Source: three-view drawing plus pictorial views. Frame: mm from the lowest corner of the part. A direction names the side the tool comes from. Coordinates: 2 decimals unless noted, no trailing zeros. Order: outer loops, then holes, each group sorted by start corner. A loop starts at its lowest first (then second) coordinate and runs counter-clockwise, first axis right, second up. Notation, with made-up numbers: (85, 76.25) -> (94, 76.25) arc R18 ccw to (94, 95.25) -> close; hole circle Ø11 at (-11.75, 37.5). An arc over 180 degrees is marked (long way). One line per question, with ' | ' between items.
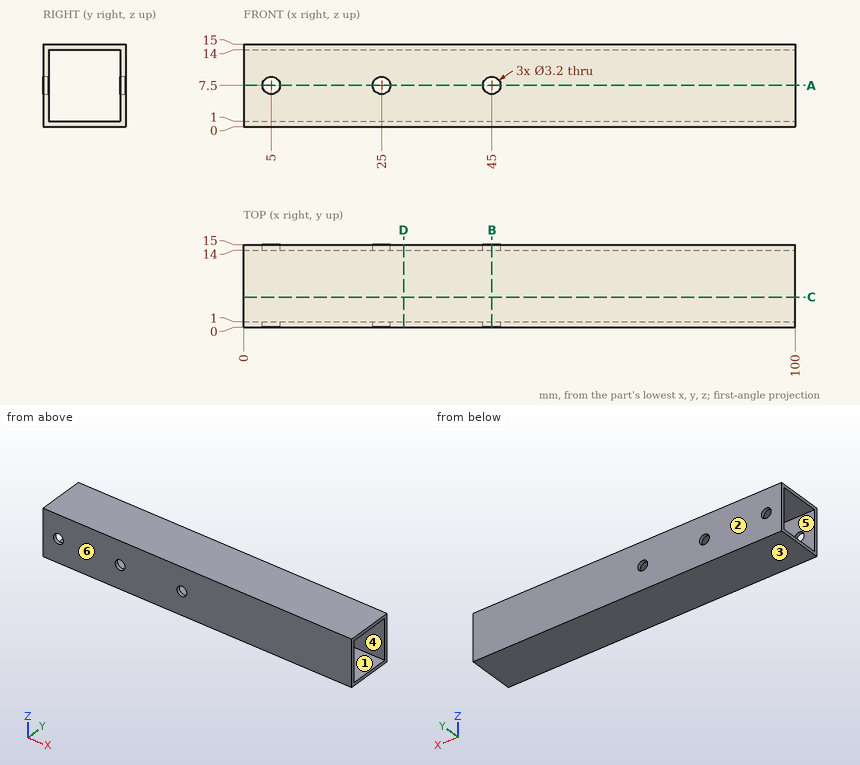
1. Access query for the marked faces 5 and 6. Directions: +Z, -Z, +X, -X, +Y, -Y. A direction counts if a zero-diameter tool reaches every point of the face in a straight line with its end or side. Return the directions, or none.
Recorded:
face 5: +X, -X | face 6: +Z, -Z, +X, -X, -Y
2. Pin query (flat end, axial travel): pin 1 Ø1.9 at (x, z) = (5, 7.5) entering from +Y; pin 2 Ø4 at (x, z) = (32.5, 3.5) entering from -Y. Return the tip coordinate at first contact, or that it passes through.
Recorded:
pin 1: passes through | pin 2: stops at y = 0
3. Ray query, line 1 (X direction, y = 0.4, z = 7.5); line 2 (Y direction, x = 71, z = 8.5). Return the intervals inside material, ascending. Write a range as [from, to].
Recorded:
line 1: x = [0, 3.4], [6.6, 23.4], [26.6, 43.4], [46.6, 100] | line 2: y = [0, 1], [14, 15]
4. Cut plane D-D, the plane x = 29. Return loops of the section in (y, z), and give its area (3 significant figures).
Recorded:
outline: (0, 0) -> (15, 0) -> (15, 15) -> (0, 15) -> close; hole (1, 1) -> (14, 1) -> (14, 14) -> (1, 14) -> close | area: 56.0 mm^2
5. Cut plane C-C, the plane y = 5.5. Return loops of the section in (x, z), and give its area (3 significant figures).
Recorded:
outline: (0, 0) -> (100, 0) -> (100, 1) -> (0, 1) -> close; (0, 14) -> (100, 14) -> (100, 15) -> (0, 15) -> close | area: 200 mm^2
6. Cut plane A-A, the plane z = 7.5. State how many separate pieces and enclosed holes the cut face has, and give its area (3 significant figures).
Recorded:
separate pieces: 8 | enclosed holes: 0 | area: 181 mm^2
7. Mould query, pull axis Z, two halves, no side actions, for the marked faces 1, 2, 3 and 4. Classes: released by +Z, released by -Z, zero draft, split by the parting line, or undercut.
Recorded:
face 1: undercut | face 2: zero draft | face 3: released by -Z | face 4: undercut
8. Cut plane B-B, the plane x = 45. Return loops of the section in (y, z), and give its area (3 significant figures).
Recorded:
outline: (0, 0) -> (15, 0) -> (15, 5.9) -> (14, 5.9) -> (14, 1) -> (1, 1) -> (1, 5.9) -> (0, 5.9) -> close; (0, 9.1) -> (1, 9.1) -> (1, 14) -> (14, 14) -> (14, 9.1) -> (15, 9.1) -> (15, 15) -> (0, 15) -> close | area: 49.6 mm^2
